Geometry: final body of the model. Coordinates: model frame, mm. A direction names the side the tool comes from. Give positions to 0.01 mm unless a question says otherwise; leave off trailing zeros. Write each loop counter-clockwise with the first axis right and the second up, starting at its lowest first coordinate (ties: lowest second). Pieces come first, ordered by that corner, then holes.
from build123d import *

# Parameters (mm, degrees)
BOX_W           = 36
BOX_H           = 36
BOX_DEPTH       = 36
SKETCH_R        = 3
POCKET_DEPTH    = 0.1
SKETCH001_R     = 3
POCKET001_DEPTH = 0.1
SKETCH002_R     = 3
POCKET002_DEPTH = 0.1
SKETCH003_R     = 3
POCKET003_DEPTH = 0.1
SKETCH004_R     = 3
POCKET004_DEPTH = 0.1
SKETCH005_R     = 3
POCKET005_DEPTH = 0.1


with BuildPart() as clue:
    # Sphere → Sphere (revolve)
    with BuildSketch(Plane.XZ):
        with BuildLine():
            ThreePointArc((0, -25), (25, 0), (0, 25))
            Line((0, 25), (0, -25))
        make_face()
    revolve(axis=Axis((0, 0, 0), (0, 0, 1)))


with BuildPart() as pocket005:
    # Box → Box (new body)
    with BuildSketch(Plane(origin=(-18, -18, -18), x_dir=(1, 0, 0), z_dir=(0, 0, 1))):
        with Locations((18, 18)):
            Rectangle(BOX_W, BOX_H)
    extrude(amount=BOX_DEPTH)

    # Common: intersect Clue
    add(clue.part, mode=Mode.INTERSECT)

    # Sketch (on Face3 of Common) → Pocket (cut)
    with BuildSketch(Plane.XY.offset(18)):
        with Locations((-8, 8)):
            Circle(SKETCH_R)
        with Locations((-8, 0)):
            Circle(SKETCH_R)
        with Locations((-8, -8)):
            Circle(SKETCH_R)
        with Locations((8, 8)):
            Circle(SKETCH_R)
        with Locations((8, 0)):
            Circle(SKETCH_R)
        with Locations((8, -8)):
            Circle(SKETCH_R)
    extrude(amount=-POCKET_DEPTH, mode=Mode.SUBTRACT)

    # Sketch001 (on Face4 of Pocket) → Pocket001 (cut)
    with BuildSketch(Plane.YZ.offset(18)):
        with Locations((-8, 8)):
            Circle(SKETCH001_R)
        with Locations((8, 8)):
            Circle(SKETCH001_R)
        with Locations((-8, -8)):
            Circle(SKETCH001_R)
        with Locations((8, -8)):
            Circle(SKETCH001_R)
        Circle(SKETCH001_R)
    extrude(amount=-POCKET001_DEPTH, mode=Mode.SUBTRACT)

    # Sketch002 (on Face6 of Pocket001) → Pocket002 (cut)
    with BuildSketch(Plane.XZ.offset(18)):
        with Locations((-8, 8)):
            Circle(SKETCH002_R)
        with Locations((-8, -8)):
            Circle(SKETCH002_R)
        with Locations((8, 8)):
            Circle(SKETCH002_R)
        with Locations((8, -8)):
            Circle(SKETCH002_R)
    extrude(amount=-POCKET002_DEPTH, mode=Mode.SUBTRACT)

    # Sketch003 (on Face7 of Pocket002) → Pocket003 (cut)
    with BuildSketch(Plane(origin=(0, 18, 0), x_dir=(-1, 0, 0), z_dir=(0, 1, 0))):
        with Locations((8, 8)):
            Circle(SKETCH003_R)
        Circle(SKETCH003_R)
        with Locations((-8, -8)):
            Circle(SKETCH003_R)
    extrude(amount=-POCKET003_DEPTH, mode=Mode.SUBTRACT)

    # Sketch004 (on Face1 of Pocket003) → Pocket004 (cut)
    with BuildSketch(Plane(origin=(-18, 0, 0), x_dir=(0, -1, 0), z_dir=(-1, 0, 0))):
        with Locations((8, 8)):
            Circle(SKETCH004_R)
        with Locations((-8, -8)):
            Circle(SKETCH004_R)
    extrude(amount=-POCKET004_DEPTH, mode=Mode.SUBTRACT)

    # Sketch005 (on Face7 of Pocket004) → Pocket005 (cut)
    with BuildSketch(Plane(origin=(0, 0, -18), x_dir=(1, 0, 0), z_dir=(0, 0, -1))):
        Circle(SKETCH005_R)
    extrude(amount=-POCKET005_DEPTH, mode=Mode.SUBTRACT)


solid = pocket005.part
Q1. Access query for faces 1 (the flat face through (-8, -17.9, -8)), 2 (the flat face through (-17.9, 8, -8)), 3 (the flat face through (17.9, 8, 8)), 4 (the flat face through (-8, -8, 17.9)). Directions: +Z, -Z, +X, -X, +Y, -Y. A direction counts if a zero-diameter tool reaches every point of the face in a straight line with its end or side. Return the directions, or none.
Filled sheet:
face 1: -Y
face 2: -X
face 3: +X
face 4: +Z
Q2. Section A-A on z = -12. Output: boundary loops of the cut face in (x, y).
Filled sheet:
outline: (-18, -12.53) arc R21.93 ccw to (-12.53, -18) - (12.53, -18) arc R21.93 ccw to (18, -12.53) - (18, 12.53) arc R21.93 ccw to (12.53, 18) - (-12.53, 18) arc R21.93 ccw to (-18, 12.53) - close
Q3. Section C-C on y = 10. Output: boundary loops of the cut face in (x, z).
Filled sheet:
outline: (-18, -14.18) arc R22.91 ccw to (-14.18, -18) - (14.18, -18) arc R22.91 ccw to (18, -14.18) - (18, -10.24) - (17.9, -10.24) - (17.9, -5.76) - (18, -5.76) - (18, 5.76) - (17.9, 5.76) - (17.9, 10.24) - (18, 10.24) - (18, 14.18) arc R22.91 ccw to (14.18, 18) - (10.24, 18) - (10.24, 17.9) - (5.76, 17.9) - (5.76, 18) - (-5.76, 18) - (-5.76, 17.9) - (-10.24, 17.9) - (-10.24, 18) - (-14.18, 18) arc R22.91 ccw to (-18, 14.18) - (-18, -5.76) - (-17.9, -5.76) - (-17.9, -10.24) - (-18, -10.24) - close
Q4. Pull-direction query (Y, two-part tool) for faces 5 (the flat face through (0, 17.9, 0)), 6 (the flat face through (8, -8, 17.9)), 7 (the flat face through (4, 0, -18)); classes: released by +Y, released by -Y, zero draft, split by the parting line, or undercut.
Filled sheet:
face 5: released by +Y
face 6: undercut
face 7: zero draft
Q5. Ray query, line 1 along Z through (x, y) = (-9.5, -10); line 2 along Z through (x, y) = (15, 10.5); line 3 along X through (y, z) = (16.5, 9). Return the intervals inside material, ascending.
Filled sheet:
line 1: z = -18 to 17.9
line 2: z = -17.02 to 17.02
line 3: x = -16.48 to 16.48
Q6. Section B-B on x = 15.5. Output: boundary loops of the cut face in (y, z), plus the area to 3 significant figures.
Filled sheet:
outline: (-18, -7.79) arc R19.62 ccw to (-7.79, -18) - (7.79, -18) arc R19.62 ccw to (18, -7.79) - (18, 7.79) arc R19.62 ccw to (7.79, 18) - (-7.79, 18) arc R19.62 ccw to (-18, 7.79) - close
area: 1,140 mm2
Q7. Pin query (flat end, axial travel): P1, Ø1.5, axis at x = -7.5, z = -6.5, coming from the -Y side; P2, Ø3, axis at y = -7, z = -8, coming from the +X side; P3, Ø5.5, axis at x = -8, y = -8, coming from the +Z side. Return the tip coordinate at first contact, or that it passes through.
Filled sheet:
P1: stops at y = -17.9
P2: stops at x = 17.9
P3: stops at z = 17.9
